Drawing for the job (mm, zero at the part's lowest x, y, z). A direction names the side the tool comes from. Coordinates: 2 decimals unless noted, no trailing zeros. Write each loop counter-clockwise with the first axis right and the second up, starting at its lowest first coordinate (ties: lowest second). Pieces come first, ordered by that corner, then holes. Notation, with made-up numbers: M -30,46.25 L -3,46.25 A22 ccw -3,75.25 Z; hole C -38,81.5 d1. An arc over 180 degrees is marked long. Put each result on its own line as item: value. Start each with the question number.
Q1. Drop flat-ended pins along their axis: pin 1 (5.5 mm diameter, centred on x = 5, y = 14, fed in from +Z); pin 2 (1.5 mm diameter, centred on y = 13, z = 3, fed in from +X); pin 3 (6.5 mm diameter, centred on x = 8.5, z = 5, fed in from +Y). Give the stop position or say it passes through.
Q2. Pull direction Y, two halves, no side cores. Call the marked faces 3, 4, 5 and 6: pulls with the +Y half, pulls with the -Y half, needs draft (parallel to the pull), parting line crosses it, or undercut.
Q3. Cut at B-B (x = 7.5). Write the cut outline in (y, z).
Q4. Cut at C-C (z = 6). Write the cut outline in (x, y).
Q5. Drill centre lines: line 1 along Z through (x, y) = (2.45, 5.9); line 2 along Y through (x, z) = (3.75, 2.75); line 3 along Y through (x, z) = (10.5, 11). Where is each one in solid material? Low to high.
Q6. Which spindle directions (+Z, -Z, +X, -X, +Y, -Y) get a long thin tool onto all of the face, cutting with end or side? Do the marked faces 1 and 2. Say none if no direction does.
Q7. Cut at A-A (y = 5.9). Write the cut outline in (x, z).
Q8. Cut at D-D (x = 13). Write the cut outline in (y, z).
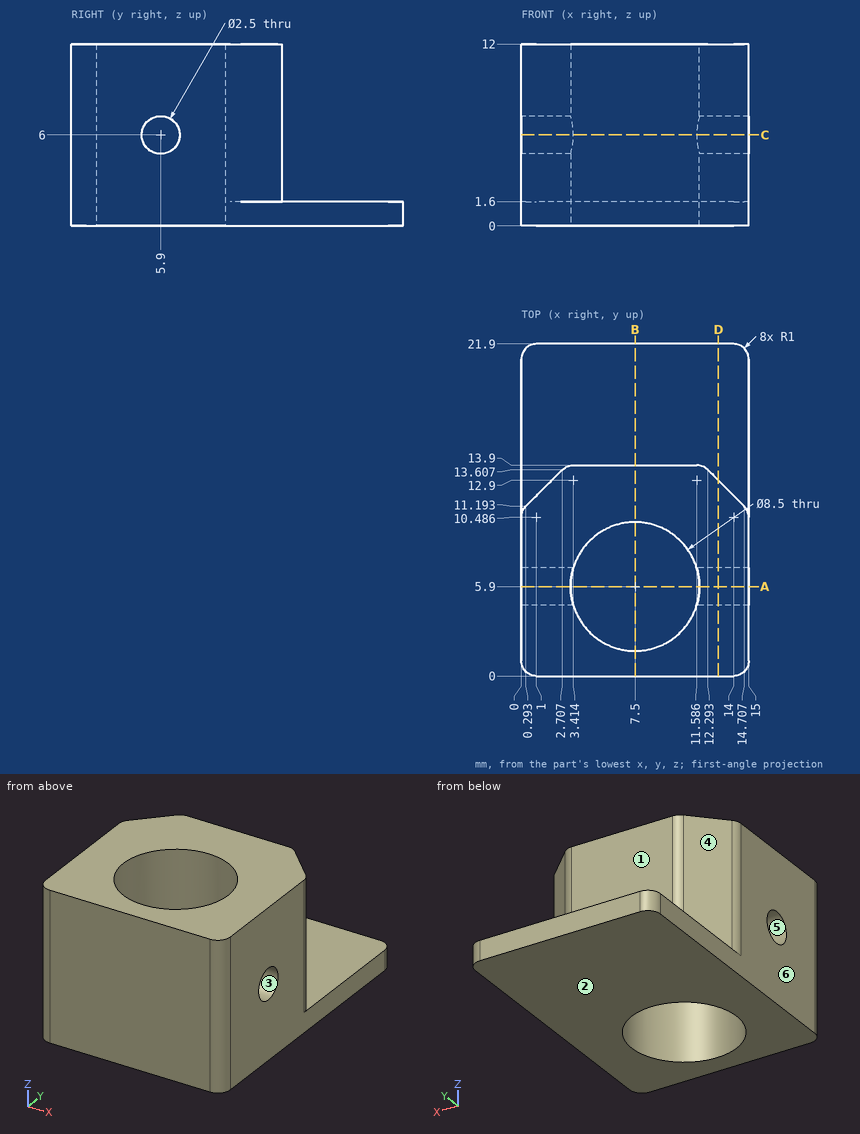
Computed values:
1. pin 1: z = 12
1. pin 2: x = 13.65
1. pin 3: y = 13.9
2. face 3: undercut
2. face 4: pulls with the +Y half
2. face 5: undercut
2. face 6: needs draft
3. outline: M 0,0 L 1.65,0 L 1.65,12 L 0,12 Z; M 10.15,0 L 21.9,0 L 21.9,1.6 L 13.9,1.6 L 13.9,12 L 10.15,12 Z
4. outline: M 0,1 A1 ccw 1,0 L 14,0 A1 ccw 15,1 L 15,4.65 L 11.56,4.65 A4.25 cw 3.44,4.65 L 0,4.65 Z; M 0,7.15 L 3.44,7.15 A4.25 cw 11.56,7.15 L 15,7.15 L 15,10.49 A1 ccw 14.71,11.19 L 12.29,13.61 A1 ccw 11.59,13.9 L 3.41,13.9 A1 ccw 2.71,13.61 L 0.29,11.19 A1 ccw 0,10.49 Z
5. line 1: 0 to 4.75, 7.25 to 12
5. line 2: 0 to 3.9, 7.9 to 13.9
5. line 3: 0 to 2.89, 8.91 to 13.9
6. face 1: +Z, +X, -X, +Y
6. face 2: -Z, +X, -X, +Y, -Y
7. outline: M 0,0 L 3.25,0 L 3.25,4.75 L 0,4.75 Z; M 0,7.25 L 3.25,7.25 L 3.25,12 L 0,12 Z; M 11.75,0 L 15,0 L 15,4.75 L 11.75,4.75 Z; M 11.75,7.25 L 15,7.25 L 15,12 L 11.75,12 Z
8. outline: M 0,0 L 21.9,0 L 21.9,1.6 L 12.9,1.6 L 12.9,12 L 0,12 Z; hole C 5.9,6 d2.5
